The listing builds one solid part. Answer for the finished solid, in the listing's coordinates (mm). Face numbers are marked on the shaded views. A direction names the side the tool comes from. Coordinates: 2 decimals unless noted, no trailing zeros. Order: outer loops, then holes, each group sorted by start corner. A loop starts at its lowest first (then second) coordinate and runs counter-clockwise, first axis right, second up. Notation, with made-up numbers: (56, 72) -> (82, 72) arc R27 cw to (82, 103) -> close; hole circle Ø3 at (52.5, 28.5). An arc over 180 degrees is marked (long way). Return JSON: item names as keys, results as strings.
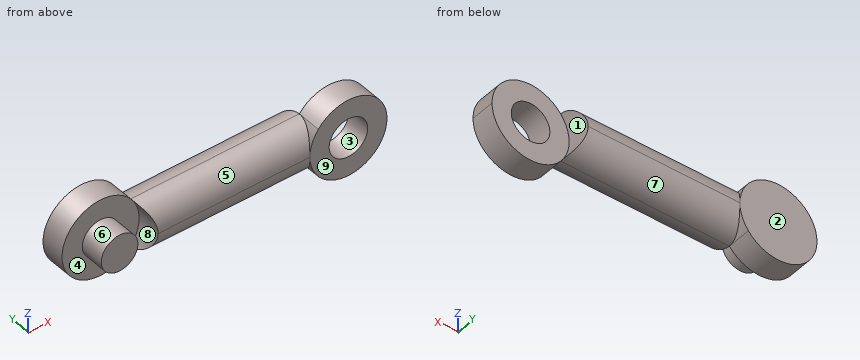
from build123d import *

# Parameters (mm, degrees)
F1_DEPTH = 6.35
F2_R     = 6.3499
F0_R     = 5.08
F3_DEPTH = 6.35
F0_R_2   = 4.826
F4_DEPTH = 6.35
F5_DEPTH = 6.35


# Not quite as in the source:
# - a fillet or chamfer is up to 0.001 mm smaller than in the source, because OpenCascade refuses the exact size


with BuildPart() as f1:
    # F0 (on Front) → F1 (new body, symmetric)
    with BuildSketch(Plane.XZ):
        with BuildLine():
            Line((22.225, 6.35), (-22.225, 6.35))
            ThreePointArc((-22.225, 6.35), (-20.5695407024, 3.3649028089), (-19.996147458, 0))
            ThreePointArc((-19.996147458, 0), (-20.5695407024, -3.3649028089), (-22.225, -6.35))
            Line((-22.225, -6.35), (22.225, -6.35))
            ThreePointArc((22.225, -6.35), (19.996147458, 0), (22.225, 6.35))
        make_face()
    extrude(amount=F1_DEPTH, both=True)

    # F2 (radius 6.35 in the source; OpenCascade refuses exactly that, so slightly less here)
    f2_edges = [f1.edges().sort_by_distance(p)[0] for p in [
        (0, -6.35, 6.35),
        (0, 6.35, 6.35),
        (0, -6.35, -6.35),
        (0, 6.35, -6.35),
    ]]
    fillet(f2_edges, radius=F2_R)

    # F0 (on Front) → F3 (join)
    with BuildSketch(Plane.XZ):
        with BuildLine():
            ThreePointArc((40.316147458, 0), (33.5210502669, 9.5866067556), (22.225, 6.35))
            Line((22.225, 6.35), (22.225, -6.35))
            ThreePointArc((22.225, -6.35), (33.5210502669, -9.5866067556), (40.316147458, 0))
        make_face()
        with Locations((30.156147458, 0)):
            Circle(F0_R, mode=Mode.SUBTRACT)
        with BuildLine():
            Line((22.225, -6.35), (22.225, 6.35))
            ThreePointArc((22.225, 6.35), (19.996147458, 0), (22.225, -6.35))
        make_face()
    extrude(amount=F3_DEPTH)

    # F0 (on Front) → F4 (join)
    with BuildSketch(Plane.XZ):
        with BuildLine():
            Line((-22.225, -6.35), (-22.225, 6.35))
            ThreePointArc((-22.225, 6.35), (-40.316147458, 0), (-22.225, -6.35))
        make_face()
        with Locations((-30.156147458, 0)):
            Circle(F0_R_2, mode=Mode.SUBTRACT)
        with BuildLine():
            ThreePointArc((-19.996147458, 0), (-20.5695407024, 3.3649028089), (-22.225, 6.35))
            Line((-22.225, 6.35), (-22.225, -6.35))
            ThreePointArc((-22.225, -6.35), (-20.5695407024, -3.3649028089), (-19.996147458, 0))
        make_face()
    extrude(amount=-F4_DEPTH)

    # F0 (on Front) → F5 (join, symmetric)
    with BuildSketch(Plane.XZ):
        with Locations((-30.156147458, 0)):
            Circle(F0_R_2)
    extrude(amount=F5_DEPTH, both=True)


solid = f1.part
1. Consider line 1 (X direction, y = -3.5, z = -1.75); line 2 (Z direction, x = 13.5, y = 0); line 3 (Z direction, x = 29.5, y = -1.5). Determine where each line is inside the solid, lowest interval first. Write a range as from..to.
Answer block:
{"line 1": "x = -34.65..-25.66, -20.15..25.39, 34.93..40.16", "line 2": "z = -6.35..6.35", "line 3": "z = -10.14..-5.04, 5.04..10.14"}
2. The part is cut by section B-B on x = 26. Give the vertices of the cut face in (y, z), and give its area (3 significant figures).
Answer block:
{"outline": "(-6.35, -9.27) -> (0, -9.27) -> (0, -2.92) -> (-6.35, -2.92) -> close; (-6.35, 2.92) -> (0, 2.92) -> (0, 9.27) -> (-6.35, 9.27) -> close", "area": "80.6 mm2"}
3. Determine the mould class of the marked faces 6, 7, 8 and 9 for opening direction Z: pulls with the +Z half, pulls with the -Z half, needs draft (parallel to the pull), parting line crosses it, or undercut.
Answer block:
{"face 6": "parting line crosses it", "face 7": "pulls with the -Z half", "face 8": "undercut", "face 9": "needs draft"}
4. For the marked faces 1, 2, 3, 4 and 5, determine the directions among +Z, -Z, +X, -X, +Y, -Y from which every point of the face is accessible in a straight line to the end or side of a thin tool.
Answer block:
{"face 1": "+X, +Y", "face 2": "+Z, -Z, +X, -X, +Y", "face 3": "+Y, -Y", "face 4": "-Y", "face 5": "+Z, -Y"}
5. The part is cut by section C-C on y = -2. Give the vertices of the cut face in (x, z) (3 decimals).
Answer block:
{"outline": "circle Ø9.652 at (-30.156, 0); (-21.977, -6.027) -> (21.977, -6.027) arc R10.16 ccw (long way) to (21.977, 6.027) -> (-21.977, 6.027) arc R10.16 cw to start; hole circle Ø10.16 at (30.156, 0)"}
6. The part is cut by section A-A on z = -0.75. Give the vertices of the cut face in (x, y), and give its area (3 significant figures).
Answer block:
{"outline": "(-40.29, 0) -> (-34.92, 0) -> (-34.92, -6.35) -> (-25.39, -6.35) -> (-25.39, 0) -> (-20.02, 0) -> (-20.02, -6.31) -> (20.02, -6.31) -> (20.02, -6.35) -> (25.13, -6.35) -> (25.13, 0) -> (20.02, 0) -> (20.02, 6.31) -> (-20.02, 6.31) -> (-20.02, 6.35) -> (-40.29, 6.35) -> close; (35.18, -6.35) -> (40.29, -6.35) -> (40.29, 0) -> (35.18, 0) -> close", "area": "759 mm2"}
7. Each of these flat-tipped pins is pushed along its axis until it touches: pin 1 Ø1 at (x, z) = (24, 5.5) entering from +Y; pin 2 Ø4 at (y, z) = (0, -7) entering from +X; pin 3 Ø6 at (x, z) = (17, -1) entering from -Y; pin 4 Ø2 at (x, y) = (-32, 2) entering from -Z. Where does it stop, or does it pass through?
Answer block:
{"pin 1": "stops at y = 0", "pin 2": "stops at x = 39", "pin 3": "stops at y = -6.35", "pin 4": "stops at z = -10.12"}
